Verification items for the finished model (mm, model axes). Face numbers are marked on the shaded views. A direction names the side the tool comes from. Coordinates: 2 decimals unless noted, no trailing zeros. Write each loop counter-clockwise with the first axis right and the second up, starting at its lowest first coordinate (ties: lowest second). Pieces come first, ordered by that corner, then holes. Notation, with made-up numbers: (-12, -13.75) -> (46, -13.75) arc R27 ccw to (46, 7.25) -> close; hole circle Ø9 at (-31, 49.5). An arc over 180 degrees is marked (long way). Answer in a Markdown table with one row per item.
```python
from build123d import *

# Parameters (mm, degrees)
SKETCH_1_R          = 32.085
EXTRUDE_1_DEPTH     = 11
SKETCH_2_R          = 34
EXTRUDE_2_DEPTH     = 1
EXTRUDE_START       = 1
SKETCH_3_R          = 34
EXTRUDE_3_DEPTH     = 1
SKETCH_4_R          = 12.5
CUT_EXTRUDE_1_DEPTH = 50.809637622
EXTRUDE_START_2     = 10
SKETCH_5_R          = 22.5
SKETCH_5_R_2        = 12.5
EXTRUDE_4_DEPTH     = 10


with BuildPart() as part:
    # 草图1 → 凸台-拉伸1 (new body)
    with BuildSketch(Plane(origin=(0, 0, 0), x_dir=(1, 0, 0), z_dir=(0, 1, 0))):
        with Locations(Location((0, 0, 0), (0, 0, 270))):
            Circle(SKETCH_1_R)
    extrude(amount=EXTRUDE_1_DEPTH)

    # 草图2 → 凸台-拉伸2 (add)
    with BuildSketch(Plane(origin=(0, 11, 0), x_dir=(1, 0, 0), z_dir=(0, 1, 0))):
        with Locations(Location((0, 0, 0), (0, 0, 270))):
            Circle(SKETCH_2_R)
    extrude(amount=EXTRUDE_2_DEPTH)

    # 草图3 → 凸台-拉伸3 (add)
    with BuildSketch(Plane.XZ.offset(EXTRUDE_START)):
        with Locations(Location((0, 0, 0), (0, 0, 90))):
            Circle(SKETCH_3_R)
    extrude(amount=-EXTRUDE_3_DEPTH)

    # 草图4 → 切除-拉伸1 (cut, through all)
    with BuildSketch(Plane(origin=(0, 12, 0), x_dir=(1, 0, 0), z_dir=(0, 1, 0))):
        with Locations(Location((0, 0, 0), (0, 0, 270))):
            Circle(SKETCH_4_R)
    extrude(amount=-CUT_EXTRUDE_1_DEPTH, mode=Mode.SUBTRACT)

    # 草图5 → 凸台-拉伸4 (add)
    with BuildSketch(Plane(origin=(0, 12, 0), x_dir=(1, 0, 0), z_dir=(0, 1, 0)).offset(EXTRUDE_START_2)):
        with Locations(Location((0, 0, 0), (0, 0, 270))):
            Circle(SKETCH_5_R)
        with Locations(Location((0, 0, 0), (0, 0, 270))):
            Circle(SKETCH_5_R_2, mode=Mode.SUBTRACT)
    extrude(amount=-EXTRUDE_4_DEPTH)


solid = part.part
```
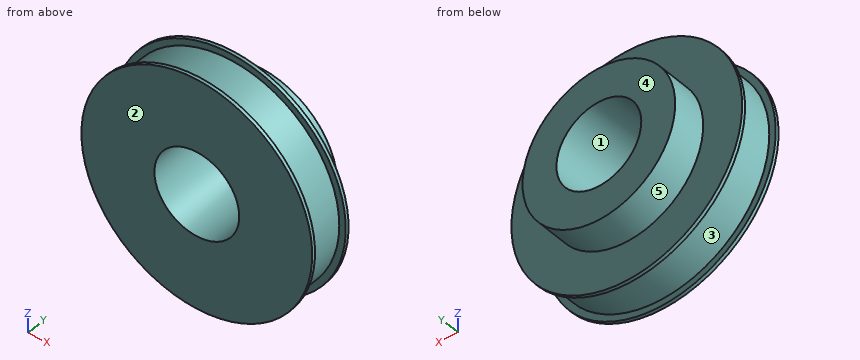
1. Go/stop test with flat-tipped pins: pin 1 (6 mm diameter, centred on y = 16, z = 17.5, fed in from -X); pin 2 (6 mm diameter, centred on y = 2.5, z = 4.5, fed in from +X); pin 3 (12 mm diameter, centred on y = 18.5, z = 6.5, fed in from +X). Record where each tip stops, or that it passes through.
Findings below:
| item | result |
|---|---|
| pin 1 | stops at x = -17.2 |
| pin 2 | stops at x = 33.88 |
| pin 3 | stops at x = 22.49 |
2. Sectioned sample at D-D, the plane x = 19.5. Record the cut outline in (y, z).
Findings below:
| item | result |
|---|---|
| outline | (-1, -27.85) -> (0, -27.85) -> (0, -25.48) -> (11, -25.48) -> (11, -27.85) -> (12, -27.85) -> (12, -11.22) -> (22, -11.22) -> (22, 11.22) -> (12, 11.22) -> (12, 27.85) -> (11, 27.85) -> (11, 25.48) -> (0, 25.48) -> (0, 27.85) -> (-1, 27.85) -> close |
3. Sectioned sample at A-A, the plane z = 0. Record the cut outline in (x, y) (3 decimals).
Findings below:
| item | result |
|---|---|
| outline | (-34, -1) -> (-12.5, -1) -> (-12.5, 22) -> (-22.5, 22) -> (-22.5, 12) -> (-34, 12) -> (-34, 11) -> (-32.085, 11) -> (-32.085, 0) -> (-34, 0) -> close; (12.5, -1) -> (34, -1) -> (34, 0) -> (32.085, 0) -> (32.085, 11) -> (34, 11) -> (34, 12) -> (22.5, 12) -> (22.5, 22) -> (12.5, 22) -> close |
4. Sectioned sample at B-B, the plane x = 0. Record the cut outline in (y, z) (3 decimals).
Findings below:
| item | result |
|---|---|
| outline | (-1, -34) -> (0, -34) -> (0, -32.085) -> (11, -32.085) -> (11, -34) -> (12, -34) -> (12, -22.5) -> (22, -22.5) -> (22, -12.5) -> (-1, -12.5) -> close; (-1, 12.5) -> (22, 12.5) -> (22, 22.5) -> (12, 22.5) -> (12, 34) -> (11, 34) -> (11, 32.085) -> (0, 32.085) -> (0, 34) -> (-1, 34) -> close |
5. Sectioned sample at C-C, the plane y = 5.5. Record the cut outline in (x, z) (3 decimals), and give its area (3 significant figures).
Findings below:
| item | result |
|---|---|
| outline | circle Ø64.17 at (0, 0); hole circle Ø25 at (0, 0) |
| area | 2,740 mm² |
6. Access from +Z, -Z, +X, -X, +Y, -Y to the whole of each face (thin tool, end or side, straight path). Record for the marked faces 4 and 5.
Findings below:
| item | result |
|---|---|
| face 4 | +Z, -Z, +X, -X, +Y |
| face 5 | +Y |
7. Material ranges on probe 1 along Y at (x, z) = (30, 11.5); probe 2 along X at (y, z) = (17.25, 0); probe 3 along Y at (x, z) = (-7.5, 28), recorded low to high. Write a range as from..to.
Findings below:
| item | result |
|---|---|
| probe 1 | y = -1..0, 11..12 |
| probe 2 | x = -22.5..-12.5, 12.5..22.5 |
| probe 3 | y = -1..12 |
8. Release check for a two-part mould opening along Z. For the marked faces 1, 2 and 3 record: released by +Z, released by -Z, zero draft, split by the parting line, or undercut.
Findings below:
| item | result |
|---|---|
| face 1 | undercut |
| face 2 | zero draft |
| face 3 | split by the parting line |
